Design review of the part built by this model. Coordinates are the model's own, in mm. A direction names the side the tool comes from. Coordinates: 2 decimals unless noted, no trailing zeros. Loops run counter-clockwise (first coordinate to the right, second up) from the corner with the lowest first, then second, coordinate; pieces in that order, holes last.
from build123d import *

# Parameters (mm, degrees)
F1_DEPTH = 350
F2_R     = 5.5
F3_DEPTH = 25


with BuildPart() as f1:
    # F0 (on Right) → F1 (new body)
    with BuildSketch(Plane.YZ):
        Polygon((0, 30), (0, 0), (40, 0), (40, 2), (2, 2), (2, 30), align=None)
    extrude(amount=F1_DEPTH)

    # F2 (on face) → F3 (cut)
    with BuildSketch(Plane.XY.offset(2)):
        with Locations((20, 21)):
            Circle(F2_R)
        with Locations((62, 20)):
            Circle(F2_R)
    extrude(amount=-F3_DEPTH, mode=Mode.SUBTRACT)


solid = f1.part
Q1. The part is to be moulded in two halves that separate along X. For faces 1 (the flat face through (350, 14, 1.7)), 2 (the cylindrical face through (56.505, 20.242, 1.014)), 3 (the flat face through (173, 21, 2)), say which applies: pulls with the +X half, pulls with the -X half, needs draft (parallel to the pull), parting line crosses it, or undercut.
Q2. Take a section at B-B, the plane x = 282. Write out the cut boundary in (y, z), then the cut area to 3 significant figures.
Q3. Clearance check with flat-ended pins moving along their axes: pin 1 Ø1 at (x, y) = (314.5, 24.5) entering from +Z; pin 2 Ø14 at (x, z) = (209.5, 15.5) entering from +Y. State where each tip first meets the part, or that it passes through.
Q4. Take a section at C-C, the plane y = 31. Write out the cut boundary in (x, z).
Q5. Take a section at A-A, the plane x = 20. Write out the cut boundary in (y, z), then the cut area to 3 significant figures.
Q6. For line 1 (Y direction, x = 20, z = 0.7); line 2 (Y direction, x = 62, z = 1.25); line 3 (Y direction, x = 275.5, z = 8), list the stretches that pass through material, from the lowest coordinate up.
Q7. Machinability: for faces 4 (the flat face through (173, 2, 16)), 5 (the flat face through (173, 0, 15)), which of the approach directions +Z, -Z, +X, -X, +Y, -Y give a long, thin tool a straight path to every point of the face, cutting with its end or side? Answer none if there is none.
Entries:
1. face 1: pulls with the +X half
1. face 2: undercut
1. face 3: needs draft
2. outline: (0, 0) - (40, 0) - (40, 2) - (2, 2) - (2, 30) - (0, 30) - close
2. area: 136 mm2
3. pin 1: stops at z = 2
3. pin 2: stops at y = 2
4. outline: (0, 0) - (350, 0) - (350, 2) - (0, 2) - close
5. outline: (0, 0) - (15.5, 0) - (15.5, 2) - (2, 2) - (2, 30) - (0, 30) - close; (26.5, 0) - (40, 0) - (40, 2) - (26.5, 2) - close
5. area: 114 mm2
6. line 1: y = 0 to 15.5, 26.5 to 40
6. line 2: y = 0 to 14.5, 25.5 to 40
6. line 3: y = 0 to 2
7. face 4: +Z, +X, -X, +Y
7. face 5: +Z, -Z, +X, -X, -Y
